Check sheet for the modelled part. Datum: model origin and axes. Units: mm. A direction names the side the tool comes from. Give positions to 0.01 mm unless a question says otherwise; leave off trailing zeros. Order: outer loops, then holes, each group sorted by start corner. A loop starts at its lowest first (then second) coordinate and runs counter-clockwise, first axis right, second up. Notation, with made-up numbers: (51, 81.5) - (89, 81.5) arc R28 ccw to (89, 108.5) - close; hole circle Ø9 at (60, 15). An arc over 180 degrees is marked (long way). Answer in a Markdown table with one row per item.
Autodesk Inventor part; units mm, degrees
ref_plane "Work Plane1" through (0, 0, 87) normal (0, 0, 1) x (1, 0, 0)
ref_plane "YZ Plane" through (0, 0, 0) normal (1, 0, 0) x (0, 1, 0)
ref_plane "XZ Plane" through (0, 0, 0) normal (0, 1, 0) x (-1, 0, 0)
sketch "Sketch4" plane through (0, 0, 0) normal (0, 0, 1) x (1, 0, 0)
  arc A0 (1.3264, -75.9884) -> (75.9884, -1.3264) centre (0, 0) ccw
  arc A1 (1.0471, -59.9909) -> (59.9909, -1.0471) centre (0, 0) ccw
  line L0 (0, -92.1462) -> (0, 0) construction
  line L1 (0, 0) -> (129.1278, 0) construction
  line L2 (0, 0) -> (106.82, -1.8646) construction
  line L3 (0, 0) -> (1.3871, -79.4693) construction
  line L4 (1.0471, -59.9909) -> (1.3264, -75.9884)
  line L5 (59.9909, -1.0471) -> (75.9884, -1.3264)
  dimension "d33" = 152
  dimension "d34" = 120
  dimension "d35" = 1
  dimension "d36" = 1
extrude "Extrusion3" add sketch "Sketch4" along normal mid plane 168
shell "Shell2" thickness 3 removed faces 1 at (4.4562, -59.8343, 28)
sketch "Sketch1" plane through (0, 0, 0) normal (0, 0, 1) x (1, 0, 0)
  circle A0 centre (0, 0) radius 77.5
  circle A1 centre (0, 0) radius 76.5
  dimension "d0" = 155
  dimension "d1" = 153
sketch "Sketch2" plane through (0, 0, 87) normal (0, 0, 1) x (1, 0, 0)
  line L0 (0, 0) -> (0, -91.1898) construction
  line L1 (0, 0) -> (8.9718, -102.5486) construction
  arc A0 (7.9909, -74.1258) -> (5.0023, -74.3873) centre (6.2752, -71.726) ccw
  line L2 (5.0023, -74.3873) -> (5.1718, -76.325)
  line L3 (7.9909, -74.1258) -> (8.1604, -76.0635)
  circle A1 centre (0, 0) radius 76.5
  arc A2 (5.1718, -76.325) -> (8.1604, -76.0635) centre (0, 0) ccw
  line L4 (7.9909, -74.1258) -> (0, 0) construction
  line L5 (0, 0) -> (5.0023, -74.3873) construction
  line L6 (0, 0) -> (93.5228, -13.1438) construction
  line L7 (0, 0) -> (97.964, 0) construction
  circle A3 centre (0, 0) radius 76.5
  line L8 (68, 0) -> (76.5, 0)
  line L9 (67.3382, -9.4638) -> (75.7555, -10.6467)
  arc A4 (67.3382, -9.4638) -> (68, 0) centre (0, 0) ccw
  point P0 (75.7555, -10.6467)
  dimension "d5" = 5
  dimension "d6" = 5.9
  dimension "d7" = 72
  dimension "d8" = 3
  dimension "d12" = 8
  dimension "d32" = 68
sketch "Sketch3" plane through (75.7555, -10.6467, 84) normal (-0.1392, -0.9903, 0) x (0.9903, -0.1392, 0)
  line L0 (-8.1618, 1) -> (0, 1)
  line L1 (0, 1) -> (0, 5)
  line L2 (0, 5) -> (-8.1618, 5)
  line L3 (-8.1618, 5) -> (-8.1618, 1)
  line L4 (0, 6) -> (0, -174) construction
  line L5 (0, -1.3495) -> (0, 7.9011) construction
  line L6 (-9.1618, 0) -> (-0.7445, 0) construction
  line L7 (-0.7445, 6) -> (-9.1618, 6) construction
  line L8 (-9.1618, 6) -> (-9.1618, 0) construction
  line L9 (-76.5, -210.3802) -> (-76.5, 44.2814)
  point P0 (-76.5, -84)
  dimension "d23" = 1
  dimension "d24" = 1
  dimension "d25" = 1
properties part number "shim_former"
(1) Cross-section at D-D, the plane y = -67. Record the cut outline in (x, z).
Geometry says:
| item | result |
|---|---|
| outline | (1.17, -84) - (35.87, -84) - (35.87, 84) - (1.17, 84) - close; hole (4.17, -81) - (28.98, -81) - (28.98, 81) - (4.17, 81) - close |
(2) Cross-section at C-C, the plane y = -12. Record the cut outline in (x, z), then the cut area to 3 significant figures.
Geometry says:
| item | result |
|---|---|
| outline | (58.79, -84) - (75.05, -84) - (75.05, 84) - (58.79, 84) - (58.79, 81) - (72.01, 81) - (72.01, -81) - (58.79, -81) - close |
| area | 590 mm² |
(3) Mould release check, pull along Y, two halves, no side actions. Record for faces 3 (the flat face through (43, -46, 81)), 4 (the cylindrical face through (52.14, -51.09, -1.13)), 5 (the flat face through (44, -47, 84)), 6 (the cylindrical face through (54.315, -53.159, -1.176)): pulls with the +Y half, pulls with the -Y half, needs draft (parallel to the pull), parting line crosses it, or undercut.
Geometry says:
| item | result |
|---|---|
| face 3 | undercut |
| face 4 | undercut |
| face 5 | needs draft |
| face 6 | pulls with the -Y half |
(4) Thickness scan on L1, parallel to Z at x = 23, y = -57.5; L2, parallel to X at y = -7.5, z = -20.5; L3, parallel to Y at x = 27.5, z = -22.5. Record the ranges inside material, lowest first.
Geometry says:
| item | result |
|---|---|
| L1 | -84 to -81, 81 to 84 |
| L2 | 72.61 to 75.63 |
| L3 | -70.85 to -67.62 |
(5) Gauge pin test, flat ends, axial feed: P1, Ø2, axis at x = 29, z = 31, coming from the -Y side; P2, Ø10, axis at x = 29.5, z = -60.5, coming from the -Y side; P3, Ø6, axis at y = -59, z = 46.5, coming from the +X side. Record the tip position at first contact, or that the pin passes through.
Geometry says:
| item | result |
|---|---|
| P1 | y = -70.65 |
| P2 | y = -71.94 |
| P3 | x = 51.38 |
(6) Cross-section at B-B, the plane z = 40.5. Record the cut outline in (x, y), then the cut area to 3 significant figures.
Geometry says:
| item | result |
|---|---|
| outline | (1.05, -59.99) - (1.33, -75.99) arc R76 ccw to (75.99, -1.33) - (59.99, -1.05) arc R60 cw to (59.86, -4.05) - (72.87, -4.27) arc R73 cw to (4.27, -72.87) - (4.05, -59.86) arc R60 cw to start |
| area | 421 mm² |
(7) Cross-section at A-A, the plane x = 69.5. Record the cut outline in (y, z).
Geometry says:
| item | result |
|---|---|
| outline | (-30.75, -84) - (-1.21, -84) - (-1.21, 84) - (-30.75, 84) - close; hole (-22.33, -81) - (-4.21, -81) - (-4.21, 81) - (-22.33, 81) - close |
(8) Access from +Z, -Z, +X, -X, +Y, -Y to the whole of each face (thin tool, end or side, straight path). Record for faces 1 (the flat face through (43, -46, -81)), 2 (the cylindrical face through (2.968, -59.927, -25.281)).
Geometry says:
| item | result |
|---|---|
| face 1 | none |
| face 2 | +Z, -Z, -X, +Y |
